Autodesk Inventor part; units mm, degrees
ref_plane "YZ Plane" through (0, 0, 0) normal (1, 0, 0) x (0, 1, 0)
ref_plane "XZ Plane" through (0, 0, 0) normal (0, 1, 0) x (-1, 0, 0)
ref_plane "XY Plane" through (0, 0, 0) normal (0, 0, 1) x (1, 0, 0)
sketch "Esboço1" plane through (0, 0, 0) normal (0, 0, 1) x (-1, 0, 0)
  circle A0 centre (0, 0) radius 23
  dimension "d0" = 46
extrude "Extrusão1" add sketch "Esboço1" along normal mid plane 70
sketch "Esboço2" plane through (0, 0, -35) normal (0, 0, -1) x (1, 0, 0)
  circle A0 centre (0, 0) radius 18
  dimension "d3" = 36
extrude "Extrusão2" add sketch "Esboço2" along normal blind 29
sketch "Esboço3" plane through (0, 0, 35) normal (0, 0, 1) x (1, 0, 0)
  circle A0 centre (0, 0) radius 18
  dimension "d6" = 36
extrude "Extrusão3" add sketch "Esboço3" along normal blind 29
chamfer "Chanfro1" distance 1 angle 45 1 edges at (-18, 0, -64)
chamfer "Chanfro2" distance 1 angle 45 3 edges at (23, 0, -35) (23, 0, 35) (-18, 0, 64)
properties material "Liga de aço"
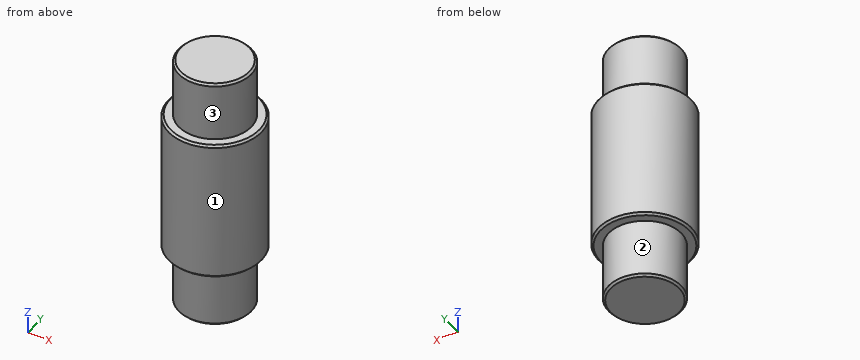
Source: CAD feature listing. Evaluate the final solid. Frame: model axes, mm. Face numbers are marked on the shaded views. A direction names the side the tool comes from. Give positions to 0.01 mm unless a question says otherwise; leave off trailing zeros. Loops run counter-clockwise (first coordinate to the right, second up) from the corner with the lowest first, then second, coordinate; pieces in that order, holes last. Notation, with made-up numbers: (50.5, 16.5) -> (72.5, 16.5) arc R13 cw to (72.5, 22.5) -> close; hole circle Ø7 at (2, -16). An arc over 180 degrees is marked (long way). Use a Markdown table: item, result. Add a question column.
(1) First-contact query: pin 1 Ø6 at (y, z) = (-15.5, 48) entering from +X; pin 2 Ø1 at (y, z) = (-12, -17) entering from -X; pin 3 Ø1.5 at (x, z) = (-6, -34.5) entering from +Y. Flat tips, straight axial feed; report the tip coordinate or a pass-through.
(2) Section query C-C (z = -53.5). Output: boundary loops of the cut face in (x, y), then the cut area to 3 significant figures.
(3) Section query D-D (z = -19). Output: boundary loops of the cut face in (x, y), then the cut area to 3 significant figures.
(4) Access query for the marked faces 1, 2 and 3. Directions: +Z, -Z, +X, -X, +Y, -Y. A direction counts if a zero-diameter tool reaches every point of the face in a straight line with its end or side. Return the directions, or none.
(5) Ray query, line 1 (X direction, y = 0.5, z = 22); line 2 (Z direction, x = 15.5, y = -15.5); line 3 (Y direction, x = 1, z = -13.5). Return the intervals inside material, ascending.
(6) Section query A-A (y = 0). Output: boundary loops of the cut face in (x, z), then the cut area to 3 significant figures.
Checked values:
| question | item | result |
|---|---|---|
| 1 | pin 1 | x = 12.95 |
| 1 | pin 2 | x = -19.92 |
| 1 | pin 3 | y = 22.35 |
| 2 | outline | circle Ø36 at (0, 0) |
| 2 | area | 1,020 mm^2 |
| 3 | outline | circle Ø46 at (0, 0) |
| 3 | area | 1,660 mm^2 |
| 4 | face 1 | +Z, -Z |
| 4 | face 2 | -Z |
| 4 | face 3 | +Z |
| 5 | line 1 | -22.99 to 22.99 |
| 5 | line 2 | -35 to 35 |
| 5 | line 3 | -22.98 to 22.98 |
| 6 | outline | (-23, -34) -> (-22, -35) -> (-18, -35) -> (-18, -63) -> (-17, -64) -> (17, -64) -> (18, -63) -> (18, -35) -> (22, -35) -> (23, -34) -> (23, 34) -> (22, 35) -> (18, 35) -> (18, 63) -> (17, 64) -> (-17, 64) -> (-18, 63) -> (-18, 35) -> (-22, 35) -> (-23, 34) -> close |
| 6 | area | 5,300 mm^2 |
